```python
from build123d import *

# Parameters (mm, degrees)
F0_W     = 1219.2
F0_H     = 1219.2
F1_DEPTH = 25.4
F2_R     = 152.4
F3_R     = 19.05
F4_DEPTH = 25.4


with BuildPart() as f1:
    # F0 (on Top) → F1 (new body)
    with BuildSketch(Plane.XY):
        Rectangle(F0_W, F0_H)
    extrude(amount=F1_DEPTH)

    # F2
    f2_edges = [f1.edges().sort_by_distance(p)[0] for p in [
        (-609.6, -609.6, 12.7),
        (609.6, -609.6, 12.7),
        (609.6, 609.6, 12.7),
        (-609.6, 609.6, 12.7),
    ]]
    fillet(f2_edges, radius=F2_R)

    # F3 (on face) → F4 (cut)
    with BuildSketch(Plane.XY.offset(25.4)):
        with Locations((-457.2, 311.15)):
            Circle(F3_R)
        with Locations((457.2, 311.15)):
            Circle(F3_R)
        with Locations((457.2, -311.15)):
            Circle(F3_R)
        with Locations((-457.2, -311.15)):
            Circle(F3_R)
    extrude(amount=-F4_DEPTH, mode=Mode.SUBTRACT)


solid = f1.part
```
For this review, take the finished solid that the model builds, in its own axes (mm). Give positions to 0.01 mm unless a question says otherwise; leave off trailing zeros. Write each loop counter-clockwise with the first axis right and the second up, starting at its lowest first coordinate (ties: lowest second). Pieces come first, ordered by that corner, then holes. Notation, with made-up numbers: M 33,-25.5 L 75,-25.5 A22 cw 75,7.5 Z; hole C 45,43.25 d11. An arc over 180 degrees is marked long. Answer as CSV lines item,"result".
1. Consider section B-B, the plane y = 311.15. Write out the cut boundary in (x, z), then the cut area to 3 significant figures.
Findings:
outline,"M -609.6,0 L -476.25,0 L -476.25,25.4 L -609.6,25.4 Z; M -438.15,0 L 438.15,0 L 438.15,25.4 L -438.15,25.4 Z; M 476.25,0 L 609.6,0 L 609.6,25.4 L 476.25,25.4 Z"
area,"29,000 mm2"
2. Consider section A-A, the plane z = 14. Write out the cut boundary in (x, y).
Findings:
outline,"M -609.6,-457.2 A152.4 ccw -457.2,-609.6 L 457.2,-609.6 A152.4 ccw 609.6,-457.2 L 609.6,457.2 A152.4 ccw 457.2,609.6 L -457.2,609.6 A152.4 ccw -609.6,457.2 Z; hole C -457.2,-311.15 d38.1; hole C -457.2,311.15 d38.1; hole C 457.2,-311.15 d38.1; hole C 457.2,311.15 d38.1"
3. Draft analysis for pull direction Y (two halves, no side actions). For faces 1 (the cylindrical face through (-566.141, 563.772, 12.878)), 2 (the cylindrical face through (-439.603, 303.854, 12.878)), 3 (the cylindrical face through (-566.141, -563.772, 12.878)), 4 (the cylindrical face through (474.797, 303.854, 12.878)), state which applies: +Y half, -Y half, draft (parallel to the pull), parting line (faces both ways), or undercut.
Findings:
face 1,"+Y half"
face 2,"undercut"
face 3,"-Y half"
face 4,"undercut"
4. Consider section C-C, the plane x = 530. Write out the cut boundary in (y, z), then the cut area to 3 significant figures.
Findings:
outline,"M -591.09,0 L 591.09,0 L 591.09,25.4 L -591.09,25.4 Z"
area,"30,000 mm2"
5. Wall thickness on line 1 (Y direction, x = -457.2, z = 6.75); line 2 (X direction, y = 302.5, z = 20.75); line 3 (X direction, y = -464, z = 3.75): over which ranges is each line inside the solid? List them lowest first.
Findings:
line 1,"y = -609.6 to -330.2, -292.1 to 292.1, 330.2 to 609.6"
line 2,"x = -609.6 to -474.17, -440.23 to 440.23, 474.17 to 609.6"
line 3,"x = -609.45 to 609.45"
6. For pin 1 (12 mm diameter, centred on x = 153.5, y = 224.5, fed in from -Z), flat-tipped, find the tip position at first contact; note if it passes through.
Findings:
pin 1,"stops at z = 0"
